Can you work these out from the drawing? Everything is in mm from the part's minimum corner. A direction names the side the tool comes from. Give positions to 0.01 mm unless a question says otherwise; leave off trailing zeros. Write each loop counter-clockwise with the first axis right and the second up, starting at its lowest first coordinate (ties: lowest second). Pieces come first, ordered by that corner, then holes. Notation, with made-up numbers: (55.25, 49) - (111.25, 49) arc R17 cw to (111.25, 62) - close; hole circle Ø6 at (-24, 12.25). An arc over 180 degrees is marked (long way). Use a Markdown table: item, result. Add a question column.
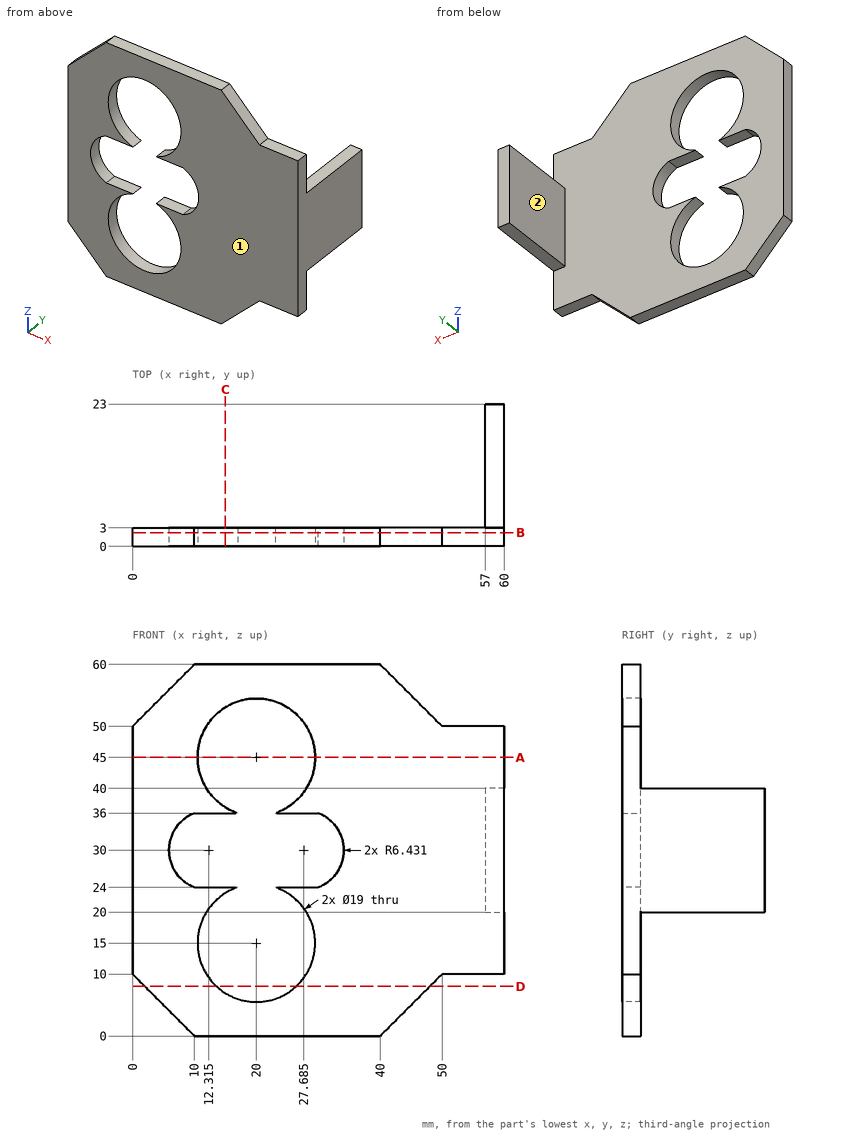
Q1. Suppose I cut it at C-C (x = 15). Please give me the cut outline in (y, z).
Q2. If I drill on probe 1 along X at (y, z) = (1.55, 45); probe 2 along Z at (x, y) = (20, 0.7); probe 3 along Y at (x, z) = (41, 28), over which ranges is the centre line in solid material (lowest first)? Write a range as [from, to].
Q3. Suppose I cut it at B-B (y = 2.25). Please give me the cut outline in (x, z) (1 decimal).
Q4. I'm going to push flat-ended pins straight in: P1, Ø0.9, axis at x = 59, y = 15.5, coming from the -Z side; P2, Ø17, axis at x = 20, z = 15, coming from the -Y side; P3, Ø1.5, axis at y = 16.5, z = 21.5, coming from the -X side; P4, Ø1.5, axis at x = 53.5, y = 2, coming from the +Z side. Where does each tip first touch, or does it pass through?
Q5. Suppose I cut it at A-A (z = 45). Please give me the cut outline in (x, y), and give its area (3 significant figures).
Q6. Suppose I cut it at D-D (z = 8). Please give me the cut outline in (x, y).
Q7. On a 3-axis mill with a long thin cutter (end or side, diameter ignored), from which of +Z, -Z, +X, -X, +Y, -Y can I reach the whole of each face in a straight line? I mean the marked faces 1 and 2. Say none if no direction works.
Derived:
| question | item | result |
|---|---|---|
| 1 | outline | (0, 0) - (3, 0) - (3, 6.92) - (0, 6.92) - close; (0, 23.08) - (3, 23.08) - (3, 24) - (0, 24) - close; (0, 36) - (3, 36) - (3, 36.92) - (0, 36.92) - close; (0, 53.08) - (3, 53.08) - (3, 60) - (0, 60) - close |
| 2 | probe 1 | [0, 10.5], [29.5, 60] |
| 2 | probe 2 | [0, 5.5], [54.5, 60] |
| 2 | probe 3 | [0, 3] |
| 3 | outline | (0, 10) - (10, 0) - (40, 0) - (50, 10) - (60, 10) - (60, 50) - (50, 50) - (40, 60) - (10, 60) - (0, 50) - close; hole (10, 24) - (17, 24) arc R9.5 ccw (long way) to (23, 24) - (30, 24) arc R6.4 ccw to (30, 36) - (23, 36) arc R9.5 ccw (long way) to (17, 36) - (10, 36) arc R6.4 ccw to start |
| 4 | P1 | z = 20 |
| 4 | P2 | through |
| 4 | P3 | x = 57 |
| 4 | P4 | z = 50 |
| 5 | outline | (0, 0) - (10.5, 0) - (10.5, 3) - (0, 3) - close; (29.5, 0) - (60, 0) - (60, 3) - (29.5, 3) - close |
| 5 | area | 123 mm² |
| 6 | outline | (2, 0) - (13.58, 0) - (13.58, 3) - (2, 3) - close; (26.42, 0) - (48, 0) - (48, 3) - (26.42, 3) - close |
| 7 | face 1 | +Z, -Z, +X, -X, -Y |
| 7 | face 2 | +Z, -Z, -X, +Y |
